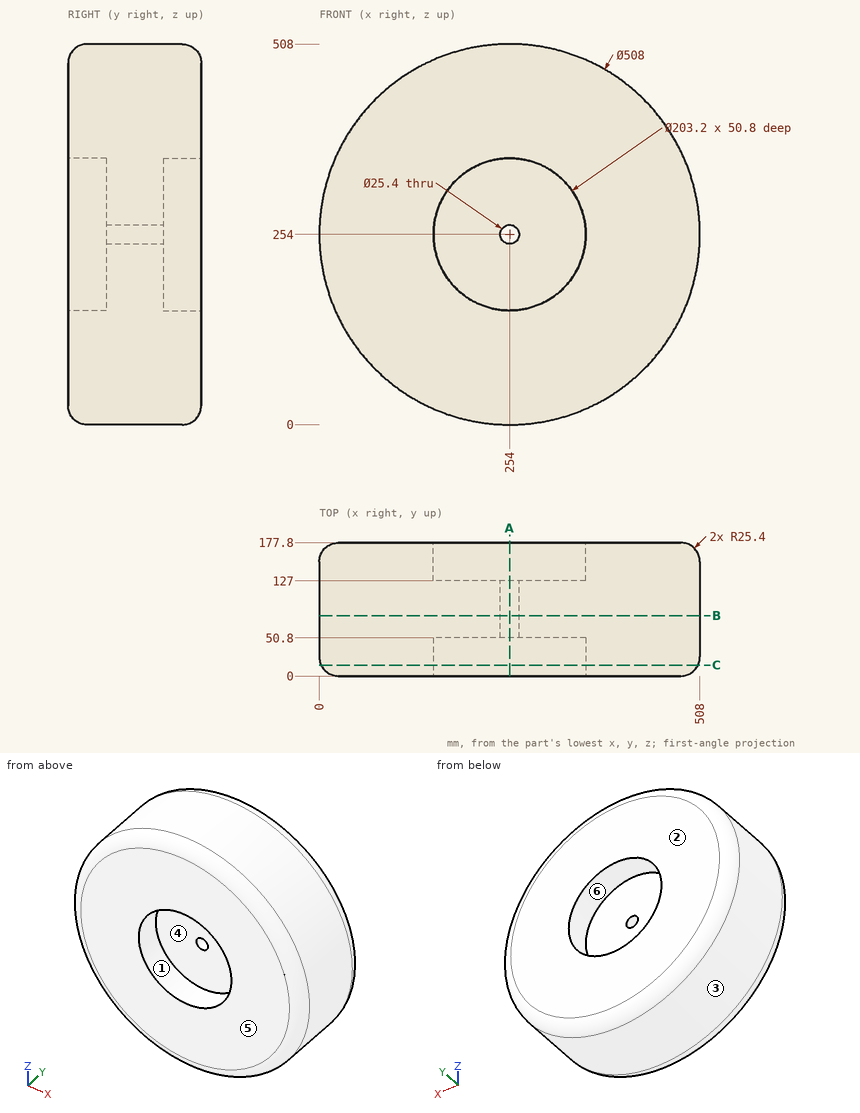
Check sheet for the drawn part. Datum: minimum x, y, z corner. Units: mm. A direction names the side the tool comes from. Give positions to 0.01 mm unless a question says otherwise; leave off trailing zeros. Order: outer loops, then holes, each group sorted by start corner. A loop starts at its lowest first (then second) coordinate and runs counter-clockwise, first axis right, second up. Notation, with made-up numbers: (-6, -40) -> (4, -40) arc R8 cw to (4, -28) -> close; hole circle Ø8 at (65, -13.5). An arc over 180 degrees is marked (long way). One line per item, written item: value.
(1) Draft check along X on the marked faces 1, 2 and 3. Enter one of: pulls with the +X half, pulls with the -X half, needs draft (parallel to the pull), parting line crosses it, or undercut.
Final values:
face 1: undercut
face 2: needs draft
face 3: parting line crosses it
(2) Tool access check on the marked faces 4, 5 and 6. Record the directions out of +Z, -Z, +X, -X, +Y, -Y that give a thin tool (end or side, any length) a straight path to the whole face; none if there is none.
Final values:
face 4: -Y
face 5: +Z, -Z, +X, -X, -Y
face 6: +Y
(3) Gauge pin test, flat ends, axial feed: pin 1 (8 mm diameter, centred on x = 332, z = 274, fed in from -Y); pin 2 (10 mm diameter, centred on y = 113, z = 373.5, fed in from +X); pin 3 (5 mm diameter, centred on y = 143, z = 403, fed in from -X). Record the tip position at first contact, or that the pin passes through.
Final values:
pin 1: y = 50.8
pin 2: x = 480.73
pin 3: x = 46.51
(4) Sectioned sample at C-C on y = 14.5. Record the cut outline in (x, z).
Final values:
outline: circle Ø503.08 at (254, 254); hole circle Ø203.2 at (254, 254)
(5) Sectioned sample at B-B on y = 80.5. Record the cut outline in (x, z).
Final values:
outline: circle Ø508 at (254, 254); hole circle Ø25.4 at (254, 254)
(6) Sectioned sample at A-A on x = 254. Record the cut outline in (y, z).
Final values:
outline: (0, 25.4) arc R25.4 ccw to (25.4, 0) -> (152.4, 0) arc R25.4 ccw to (177.8, 25.4) -> (177.8, 152.4) -> (127, 152.4) -> (127, 241.3) -> (50.8, 241.3) -> (50.8, 152.4) -> (0, 152.4) -> close; (0, 355.6) -> (50.8, 355.6) -> (50.8, 266.7) -> (127, 266.7) -> (127, 355.6) -> (177.8, 355.6) -> (177.8, 482.6) arc R25.4 ccw to (152.4, 508) -> (25.4, 508) arc R25.4 ccw to (0, 482.6) -> close
(7) Scan lines: line 1 along Z through (x, y) = (249, 31.5); line 2 along Z through (x, y) = (254, 138); line 3 along X through (y, z) = (27.5, 216). Record each from-to range of solid material in increasing order. Write a range as [from, to].
Final values:
line 1: [0.05, 152.52], [355.48, 507.95]
line 2: [0, 152.4], [355.6, 508]
line 3: [2.86, 159.77], [348.23, 505.14]
